Input: part model. Units: mm. Frame: model coordinates. Coordinates: 2 decimals unless noted, no trailing zeros. Answer as CSV lines item,"result".
from build123d import *

# Parameters (mm, degrees)
SKETCH1_W                                         = 45.745826238
SKETCH1_H                                         = 49.9872
BOSS_EXTRUDE1_DEPTH                               = 4.7625
CSK_FOR_6_FLAT_HEAD_MACHINE_SCREW_100_D           = 3.6576
CSK_FOR_6_FLAT_HEAD_MACHINE_SCREW_100_CSINK_D     = 9.4701106
CSK_FOR_6_FLAT_HEAD_MACHINE_SCREW_100_CSINK_ANGLE = 100
SKETCH8_R                                         = 1.3589
CUT_EXTRUDE1_DEPTH                                = 5.7625


with BuildPart() as part:
    # Sketch1 → Boss-Extrude1 (new body)
    with BuildSketch(Plane(origin=(0, -2000, 0), x_dir=(1, 0, 0), z_dir=(0, 1, 0))):
        with Locations((-1550.959562055, 2948.348659299)):
            Rectangle(SKETCH1_W, SKETCH1_H)
    extrude(amount=BOSS_EXTRUDE1_DEPTH)

    # CSK for #6 Flat Head Machine Screw (100)8 (through all)
    with Locations(Plane(origin=(-1560.230562055, -1995.2375, -2968.668659299), x_dir=(0, 0, 1), z_dir=(0, 1, 0))):
        with Locations((0, 0), (40.64, 0), (40.64, 18.542), (0, 18.542)):
            CounterSinkHole(CSK_FOR_6_FLAT_HEAD_MACHINE_SCREW_100_D / 2, CSK_FOR_6_FLAT_HEAD_MACHINE_SCREW_100_CSINK_D / 2, counter_sink_angle=CSK_FOR_6_FLAT_HEAD_MACHINE_SCREW_100_CSINK_ANGLE)

    # Sketch8 → Cut-Extrude1 (cut, through all)
    with BuildSketch(Plane.XZ.offset(2000)):
        with Locations((-1541.684253717, -2954.236887357)):
            Circle(SKETCH8_R)
        with Locations((-1560.226253717, -2954.236887357)):
            Circle(SKETCH8_R)
        with Locations((-1571.277192756, -2941.714687357)):
            Circle(SKETCH8_R)
        with Locations((-1530.633314678, -2941.714687357)):
            Circle(SKETCH8_R)
    extrude(amount=-CUT_EXTRUDE1_DEPTH, mode=Mode.SUBTRACT)


solid = part.part
1. Ray query, line 1 along X through (y, z) = (-1997.15, -2967); line 2 along Z through (x, y) = (-1559.5, -1997.9); line 3 along X through (y, z) = (-1998.2, -2927). Return the intervals inside material, ascending.
Findings:
line 1,"x = -1573.83 to -1562.03, -1558.43 to -1543.49, -1539.89 to -1528.09"
line 2,"z = -2973.34 to -2970.35, -2966.99 to -2955.39, -2953.09 to -2929.71, -2926.35 to -2923.36"
line 3,"x = -1573.83 to -1561.74, -1558.72 to -1543.2, -1540.18 to -1528.09"
2. Cut plane A-A (y = -1996.8). State how many separate pieces and enclosed holes the cut face has, plus the area to 3 significant figures.
Findings:
separate pieces,"1"
enclosed holes,"8"
area,"2,160 mm2"
3. Mould query, pull axis Z, two halves, no side actions, for faces 1 (the face through (-1551, -1998, -2973.342)), 2 (the face through (-1541.097, -1997.558, -2970.548)), 3 (the face through (-1573.832, -1998, -2948)), 4 (the face through (-1541.61, -1998.85, -2926.2)). Classes: released by +Z, released by -Z, zero draft, split by the parting line, or undercut.
Findings:
face 1,"released by -Z"
face 2,"undercut"
face 3,"zero draft"
face 4,"undercut"
